Part model, mm, in its own coordinate system. Coordinates: 2 decimals unless noted, no trailing zeros. Write each loop counter-clockwise with the first axis right and the second up, starting at its lowest first coordinate (ties: lowest second). Pieces come first, ordered by that corner, then holes. Notation, with made-up numbers: (-13, -30.75) -> (39, -30.75) arc R10 ccw to (39, -26.75) -> close; hole circle Ø5 at (-40, 68). An arc over 180 degrees is marked (long way). Write item = value, one per line. Start each with the question number.
Q1. Band-saw the part on C-C, the plane x = 3. List the corners of the cut face in (y, z).
Q2. Band-saw the part on B-B, the plane x = 57.5. List the corners of the cut face in (y, z).
Q3. Band-saw the part on D-D, the plane y = 1.5. Give the number of separate pieces and of enclosed holes in the cut face, plus the area to 3 significant figures.
Q4. Probe line 1 (X direction, y = 2.5, z = 22.5); line 2 (X direction, y = 0.25, z = -21); line 3 (X direction, y = 2, z = -19). List the from-to ranges inside material, lowest first.
Q5. Band-saw the part on A-A, the plane z = -11. List the corners of the cut face in (x, y).
Q6. Pin check, flat tips, straight feed: P1, Ø1, axis at y = 1, z = 11, coming from the +X side; P2, Ø12, axis at x = 2, z = 14, coming from the -Y side; P3, Ø1.6, axis at y = 1, z = -13.5, coming from the -X side. Stop position of each tip, or through.
from build123d import *

# Parameters (mm, degrees)
SKETCH_1_W          = 100
SKETCH_1_H          = 60
EXTRUDE_1_DEPTH     = 3.2
SKETCH_2_R          = 12.5
SKETCH_2_R_2        = 1.6
SKETCH_2_R_3        = 1.5
SKETCH_2_R_4        = 5.75
CUT_EXTRUDE_1_DEPTH = 3.2
FILLET_1_R          = 2
FILLET_2_R          = 1


with BuildPart() as part:
    # 草图1 → 凸台-拉伸1 (new body)
    with BuildSketch(Plane(origin=(0, 0, 0), x_dir=(1, 0, 0), z_dir=(0, 1, 0))):
        Polygon((-57.5, -15), (-60.328427125, -15), (-65, -15), (-65, -30), (-50, -30), (-50, -15), align=None)
        Rectangle(SKETCH_1_W, SKETCH_1_H)
        Polygon((-50, -7.5), (-50, -4.671572875), (-60.328427125, -15), (-57.5, -15), align=None)
        Polygon((65, -15), (60.328427125, -15), (57.5, -15), (50, -15), (50, -30), (65, -30), align=None)
        Polygon((60.328427125, -15), (50, -4.671572875), (50, -7.5), (57.5, -15), align=None)
    extrude(amount=EXTRUDE_1_DEPTH)

    # 草图2 → 切除-拉伸1 (cut)
    with BuildSketch(Plane(origin=(0, 3.2, 0), x_dir=(1, 0, 0), z_dir=(0, 1, 0))):
        with Locations(Location((0, -9.443650814, 0), (0, 0, 270))):
            Circle(SKETCH_2_R)
        with Locations(Location((15.556349186, -25, 0), (0, 0, 270))):
            Circle(SKETCH_2_R_2)
        with Locations(Location((15.556349186, 6.112698372, 0), (0, 0, 270))):
            Circle(SKETCH_2_R_2)
        with Locations(Location((-15.556349186, 6.112698372, 0), (0, 0, 270))):
            Circle(SKETCH_2_R_2)
        with Locations(Location((-15.556349186, -25, 0), (0, 0, 270))):
            Circle(SKETCH_2_R_2)
        with Locations(Location((-47.5, 20, 0), (0, 0, 270))):
            Circle(SKETCH_2_R_3)
        with Locations(Location((-47.5, -20, 0), (0, 0, 270))):
            Circle(SKETCH_2_R_3)
        with Locations(Location((47.5, -20, 0), (0, 0, 270))):
            Circle(SKETCH_2_R_3)
        with Locations(Location((47.5, 20, 0), (0, 0, 270))):
            Circle(SKETCH_2_R_3)
        with Locations(Location((-57.5, -22.5, 0), (0, 0, 270))):
            Circle(SKETCH_2_R_4)
        with Locations(Location((57.5, -22.5, 0), (0, 0, 270))):
            Circle(SKETCH_2_R_4)
        with Locations(Location((30, 19, 0), (0, 0, 270))):
            Circle(SKETCH_2_R_3)
        with Locations(Location((30, 11, 0), (0, 0, 270))):
            Circle(SKETCH_2_R_3)
        with Locations(Location((-30, 11, 0), (0, 0, 270))):
            Circle(SKETCH_2_R_3)
        with Locations(Location((-30, 19, 0), (0, 0, 270))):
            Circle(SKETCH_2_R_3)
        with Locations(Location((30, -11, 0), (0, 0, 270))):
            Circle(SKETCH_2_R_3)
        with Locations(Location((30, -19, 0), (0, 0, 270))):
            Circle(SKETCH_2_R_3)
        with Locations(Location((-30, -19, 0), (0, 0, 270))):
            Circle(SKETCH_2_R_3)
        with Locations(Location((-30, -11, 0), (0, 0, 270))):
            Circle(SKETCH_2_R_3)
        with Locations(Location((-28.065, 27, 0), (0, 0, 270))):
            Circle(SKETCH_2_R_3)
        with Locations(Location((28.065, 27, 0), (0, 0, 270))):
            Circle(SKETCH_2_R_3)
        with Locations(Location((-28.065, -16.18, 0), (0, 0, 270))):
            Circle(SKETCH_2_R_3)
        with Locations(Location((28.065, -16.18, 0), (0, 0, 270))):
            Circle(SKETCH_2_R_3)
        with Locations(Location((-28.769, -27.5, 0), (0, 0, 270))):
            Circle(SKETCH_2_R_3)
        with Locations(Location((28.769, -27.5, 0), (0, 0, 270))):
            Circle(SKETCH_2_R_3)
        with Locations(Location((-36.769, -22.5, 0), (0, 0, 270))):
            Circle(SKETCH_2_R_3)
        with Locations(Location((36.769, -22.5, 0), (0, 0, 270))):
            Circle(SKETCH_2_R_3)
    extrude(amount=-CUT_EXTRUDE_1_DEPTH, mode=Mode.SUBTRACT)

    # 圆角1
    fillet_1_edges = [part.edges().sort_by_distance(p)[0] for p in [
        (-60.328427125, 1.6, 15),
        (-50, 1.6, 4.671572875),
        (-50, 1.6, -30),
        (50, 1.6, -30),
        (50, 1.6, 4.671572875),
        (60.328427125, 1.6, 15),
        (65, 1.6, 15),
        (65, 1.6, 30),
        (-65, 1.6, 30),
        (-65, 1.6, 15),
    ]]
    fillet(fillet_1_edges, radius=FILLET_1_R)

    # 圆角2
    fillet_2_edges = [part.edges().sort_by_distance(p)[0] for p in [
        (-57.5, 1.6, 15),
        (-50, 1.6, 15),
        (-50, 1.6, 7.5),
        (50, 1.6, 7.5),
        (50, 1.6, 15),
        (57.5, 1.6, 15),
    ]]
    fillet(fillet_2_edges, radius=FILLET_2_R)


solid = part.part
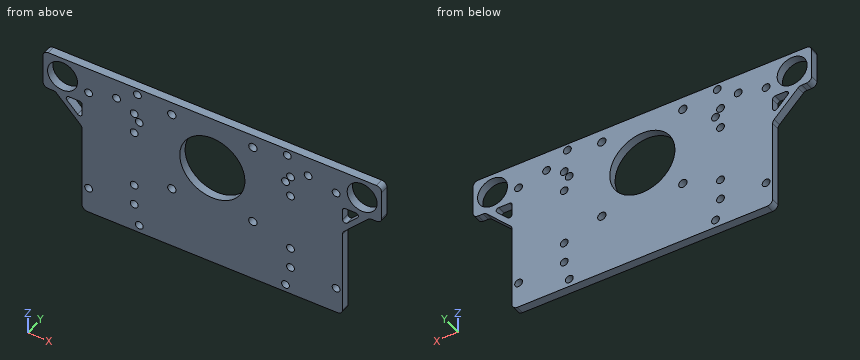
Ans:
q1.outline = (0, -30) -> (3.2, -30) -> (3.2, -2.69) -> (0, -2.69) -> close; (0, 21.58) -> (3.2, 21.58) -> (3.2, 30) -> (0, 30) -> close
q2.outline = (0, 12.17) -> (3.2, 12.17) -> (3.2, 16.75) -> (0, 16.75) -> close; (0, 28.25) -> (3.2, 28.25) -> (3.2, 30) -> (0, 30) -> close
q3.separate_pieces = 1
q3.enclosed_holes = 29
q3.area = 5,630 mm2
q4.line_1 = -65 to -63.25, -51.75 to -38.27, -35.27 to 35.27, 38.27 to 51.75, 63.25 to 65
q4.line_2 = -50 to -48.62, -46.38 to 46.38, 48.62 to 50
q4.line_3 = -50 to -48.62, -46.38 to -31.5, -28.5 to 28.5, 31.5 to 46.38, 48.62 to 50
q5.outline = (-50, 0) -> (-31.5, 0) -> (-31.5, 3.2) -> (-50, 3.2) -> close; (-28.5, 0) -> (28.5, 0) -> (28.5, 3.2) -> (-28.5, 3.2) -> close; (31.5, 0) -> (50, 0) -> (50, 3.2) -> (31.5, 3.2) -> close
q6.P1 = 56.83
q6.P2 = through
q6.P3 = -50
